from build123d import *

# Parameters (mm, degrees)
F0_W      = 9
F0_H      = 10
F0_W_2    = 44
F0_H_2    = 16
F0_W_3    = 7
F0_R      = 1
F1_DEPTH  = 0.5
F3_R      = 0.5
F3_W      = 0.3535533906
F3_H      = 10
F4_DEPTH  = 0.5
F6_R      = 0.5
F6_W      = 0.3535533906
F6_H      = 10
F7_DEPTH  = 0.5
F8_R      = 1.25
F9_DEPTH  = 0.5
F10_R     = 1.25
F11_DEPTH = 0.5
F12_DEPTH = 0.5
F14_DEPTH = 15
F13_W     = 2
F13_H     = 14.5
F15_DEPTH = 1
F16_W     = 2
F16_H     = 1
F17_DEPTH = 1
F18_W     = 1
F18_H     = 29.75
F19_DEPTH = 6.5
F21_D     = 2.5
F21_DEPTH = 8
F21_TIP   = 0.7510757738
F23_DEPTH = 1
F25_DEPTH = 1
F26_R     = 1.25
F27_DEPTH = 1
F28_W     = 5
F28_H     = 1
F29_DEPTH = 5
F30_DEPTH = 14.25
F31_W     = 5
F31_H     = 4
F31_H_2   = 1
F32_DEPTH = 1
F34_DEPTH = 0.5
F35_W     = 1
F35_H     = 42
F36_DEPTH = 0.5
F38_DEPTH = 0.5
F39_W     = 0.5
F39_H     = 42
F39_W_2   = 1
F40_DEPTH = 0.5


# Not quite as in the source:
# - a feature of the source that left no trace in its solid (it failed there, or was rolled back) is left out
# - a feature names something its author has since deleted; it is built from what else it names


with BuildPart() as f1:
    # F0 (on Front) → F1 (new body)
    with BuildSketch(Plane.XZ):
        with Locations((-25.5, 0)):
            Rectangle(F0_W, F0_H)
        with Locations((1, 13)):
            Rectangle(F0_W_2, F0_H_2)
        with Locations((1, 0)):
            Rectangle(F0_W_2, F0_H)
        with Locations((26.5, 0)):
            Rectangle(F0_W_3, F0_H)
        with Locations((1, -13)):
            Rectangle(F0_W_2, F0_H_2)
        with Locations((1, -13)):
            Circle(F0_R, mode=Mode.SUBTRACT)
    extrude(amount=F1_DEPTH)

    # F3 (on face) → F4 (join)
    with BuildSketch(Plane(origin=(15, 15, 0), x_dir=(0.7071067812, -0.7071067812, 0), z_dir=(-0.7071067812, -0.7071067812, 0))):
        with BuildLine():
            Line((21.5667568262, 5), (21.5667568262, -5))
            Line((21.5667568262, -5), (32.2132034356, -5))
            ThreePointArc((32.2132034356, -5), (32.9203102168, -4.7071067812), (33.2132034356, -4))
            Line((33.2132034356, -4), (33.2132034356, 4))
            ThreePointArc((33.2132034356, 4), (32.9203102168, 4.7071067812), (32.2132034356, 5))
            Line((32.2132034356, 5), (21.5667568262, 5))
        make_face()
        with Locations((23.2132034356, -2)):
            Circle(F3_R, mode=Mode.SUBTRACT)
        with Locations((23.2132034356, 0)):
            Circle(F3_R, mode=Mode.SUBTRACT)
        with Locations((23.2132034356, 2)):
            Circle(F3_R, mode=Mode.SUBTRACT)
        with Locations((21.3899801309, 0)):
            Rectangle(F3_W, F3_H)
    extrude(amount=F4_DEPTH)

    # F6 (on face) → F7 (join)
    with BuildSketch(Plane(origin=(-15, 15, 0), x_dir=(0.7071067812, 0.7071067812, 0), z_dir=(0.7071067812, -0.7071067812, 0))):
        with BuildLine():
            Line((-21.5667568262, -5), (-21.5667568262, 5))
            Line((-21.5667568262, 5), (-32.2132034356, 5))
            ThreePointArc((-32.2132034356, 5), (-32.9203102168, 4.7071067812), (-33.2132034356, 4))
            Line((-33.2132034356, 4), (-33.2132034356, -4))
            ThreePointArc((-33.2132034356, -4), (-32.9203102168, -4.7071067812), (-32.2132034356, -5))
            Line((-32.2132034356, -5), (-21.5667568262, -5))
        make_face()
        with Locations((-22.2132034356, -2)):
            Circle(F6_R, mode=Mode.SUBTRACT)
        with Locations((-22.2132034356, 0)):
            Circle(F6_R, mode=Mode.SUBTRACT)
        with Locations((-22.2132034356, 2)):
            Circle(F6_R, mode=Mode.SUBTRACT)
        with Locations((-21.3899801309, 0)):
            Rectangle(F6_W, F6_H)
    extrude(amount=F7_DEPTH)

    # F8 (on face) → F9 (join)
    with BuildSketch(Plane(origin=(15, 15, 0), x_dir=(-0.7071067812, 0.7071067812, 0), z_dir=(0.7071067812, 0.7071067812, 0))):
        with Locations((-30.7632034356, 0)):
            Circle(F8_R)
    extrude(amount=F9_DEPTH)

    # F10 (on face) → F11 (join)
    with BuildSketch(Plane(origin=(-15, 15, 0), x_dir=(-0.7071067812, -0.7071067812, 0), z_dir=(-0.7071067812, 0.7071067812, 0))):
        with Locations((30.7632034356, 0)):
            Circle(F10_R)
    extrude(amount=F11_DEPTH)

    # F0 (on Front) → F12 (join)
    with BuildSketch(Plane.XZ):
        with Locations((1, 13)):
            Rectangle(F0_W_2, F0_H_2)
        with Locations((1, -13)):
            Rectangle(F0_W_2, F0_H_2)
        with Locations((1, -13)):
            Circle(F0_R, mode=Mode.SUBTRACT)
    extrude(amount=F12_DEPTH)

    # F0 (on Front) → F14 (join)
    with BuildSketch(Plane.XZ):
        with Locations((1, -13)):
            Circle(F0_R)
    extrude(amount=F14_DEPTH)

    # F13 (on face) → F15 (join)
    with BuildSketch(Plane(origin=(0, 0, -21), x_dir=(1, 0, 0), z_dir=(0, 0, -1))):
        with Locations((-20, 7.75)):
            Rectangle(F13_W, F13_H)
        with Locations((22, 7.75)):
            Rectangle(F13_W, F13_H)
    extrude(amount=-F15_DEPTH)

    # F16 (on face) → F17 (join)
    with BuildSketch(Plane.XZ.offset(15)):
        with BuildLine():
            Line((-19, -21), (-21, -21))
            Line((-21, -21), (-21, -42.75))
            Line((-21, -42.75), (23, -42.75))
            Line((23, -42.75), (23, -21))
            Line((23, -21), (21, -21))
            Line((21, -21), (21, -20))
            Line((21, -20), (23, -20))
            Line((23, -20), (23, -13))
            Line((23, -13), (2, -13))
            ThreePointArc((2, -13), (1, -14), (0, -13))
            Line((0, -13), (-21, -13))
            Line((-21, -13), (-21, -20))
            Line((-21, -20), (-19, -20))
            Line((-19, -20), (-19, -21))
        make_face()
        with Locations((-20, -20.5)):
            Rectangle(F16_W, F16_H)
        with BuildLine():
            ThreePointArc((2, -13), (1, -12), (0, -13))
            Line((0, -13), (2, -13))
        make_face()
        with BuildLine():
            Line((2, -13), (0, -13))
            ThreePointArc((0, -13), (1, -14), (2, -13))
        make_face()
        with Locations((22, -20.5)):
            Rectangle(F16_W, F16_H)
    extrude(amount=F17_DEPTH)

    # F18 (on face) → F19 (join)
    with BuildSketch(Plane.XZ.offset(16)):
        with Locations((1, -27.875)):
            Rectangle(F18_W, F18_H)
    extrude(amount=F19_DEPTH)

    # F21
    with Locations(Plane.YZ.offset(1.5)):
        with Locations((-19.25, -39)):
            Hole(F21_D / 2, depth=F21_DEPTH)
            with Locations((0, 0, -(F21_DEPTH + F21_TIP / 2))):  # 118° drill point
                Cone(0, F21_D / 2, F21_TIP, mode=Mode.SUBTRACT)

    # F22 (on face) → F23 (join)
    with BuildSketch(Plane(origin=(0, 0, -42.75), x_dir=(1, 0, 0), z_dir=(0, 0, -1))):
        Polygon((-21, 15), (23, 15), (23, 16), (1.5, 16), (1.5, 22.5), (0.5, 22.5), (0.5, 16), (-21, 16), align=None)
    extrude(amount=F23_DEPTH)

    # F22 (on face) → F25 (join)
    with BuildSketch(Plane(origin=(0, 0, -42.75), x_dir=(1, 0, 0), z_dir=(0, 0, -1))):
        Polygon((1.5, 16), (23, 16), (23, 51.5), (18, 51.5), (18, 52.5), (23, 52.5), (23, 53), (23, 90), (-21, 90), (-21, 52.5), (-16, 52.5), (-16, 51.5), (-21, 51.5), (-21, 16), (0.5, 16), (0.5, 22.5), (1.5, 22.5), align=None)
        Polygon((-21, 15), (23, 15), (23, 16), (1.5, 16), (1.5, 22.5), (0.5, 22.5), (0.5, 16), (-21, 16), align=None)
    extrude(amount=F25_DEPTH)

    # F26 (on face) → F27 (join)
    with BuildSketch(Plane.XZ.offset(90)):
        Polygon((-16, -43.75), (-21, -43.75), (-21, -58), (-21, -70.1), (-16, -70.1), align=None)
        with Locations((-18.5, -67.075)):
            Circle(F26_R, mode=Mode.SUBTRACT)
        Polygon((23, -43.75), (18, -43.75), (18, -70.1), (23, -70.1), (23, -58), align=None)
        with Locations((20.5, -67.075)):
            Circle(F26_R, mode=Mode.SUBTRACT)
    extrude(amount=-F27_DEPTH)

    # F28 (on face) → F29 (join)
    with BuildSketch(Plane(origin=(0, -89, 0), x_dir=(-1, 0, 0), z_dir=(0, 1, 0))):
        with Locations((18.5, -57.5)):
            Rectangle(F28_W, F28_H)
        with Locations((-20.5, -57.5)):
            Rectangle(F28_W, F28_H)
    extrude(amount=F29_DEPTH)

    # F22 (on face) → F30 (join)
    with BuildSketch(Plane(origin=(0, 0, -42.75), x_dir=(1, 0, 0), z_dir=(0, 0, -1))):
        Polygon((-21, 52), (-21, 51.5), (-16, 51.5), (-16, 52.5), (-21, 52.5), align=None)
        Polygon((18, 51.5), (23, 51.5), (23, 52), (23, 52.5), (18, 52.5), align=None)
    extrude(amount=F30_DEPTH)

    # F31 (on face) → F32 (join)
    with BuildSketch(Plane(origin=(0, 0, -57), x_dir=(1, 0, 0), z_dir=(0, 0, -1))):
        with Locations((20.5, 49.5)):
            Rectangle(F31_W, F31_H)
        with Locations((20.5, 52)):
            Rectangle(F31_W, F31_H_2)
        with Locations((-18.5, 49.5)):
            Rectangle(F31_W, F31_H)
        with Locations((-18.5, 52)):
            Rectangle(F31_W, F31_H_2)
    extrude(amount=F32_DEPTH)

    # F33 (on face) → F34 (join)
    with BuildSketch(Plane.YZ.offset(23)):
        Polygon((0, 21), (0, 5), (0, -5), (0, -21), (1.5, -21), (1.5, 21), align=None)
    extrude(amount=-F34_DEPTH)

    # F35 (on face) → F36 (join)
    with BuildSketch(Plane(origin=(0, 1.5, 0), x_dir=(-1, 0, 0), z_dir=(0, 1, 0))):
        with Locations((-22, 0)):
            Rectangle(F35_W, F35_H)
    extrude(amount=-F36_DEPTH)

    # F37 (on face) → F38 (join)
    with BuildSketch(Plane(origin=(-21, 0, 0), x_dir=(0, -1, 0), z_dir=(-1, 0, 0))):
        Polygon((-1.5, -21), (0, -21), (0, -5), (0, 21), (-1.5, 21), align=None)
    extrude(amount=-F38_DEPTH)

    # F39 (on face) → F40 (join)
    with BuildSketch(Plane(origin=(0, 1.5, 0), x_dir=(-1, 0, 0), z_dir=(0, 1, 0))):
        with Locations((20.75, 0)):
            Rectangle(F39_W, F39_H)
        with Locations((20, 0)):
            Rectangle(F39_W_2, F39_H)
    extrude(amount=F40_DEPTH)


solid = f1.part
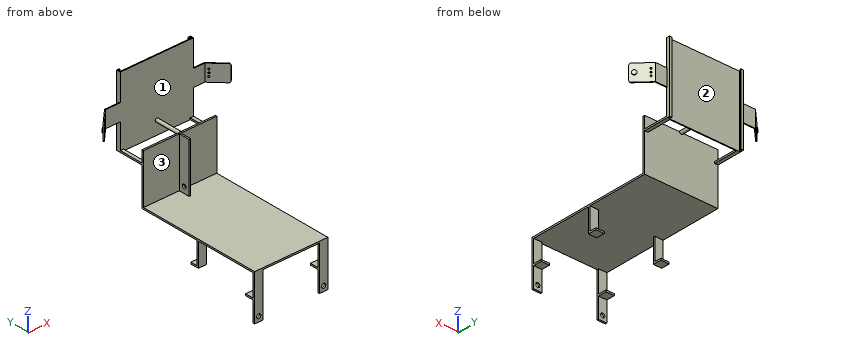
The listing builds one solid part. Answer for the finished solid, in the listing's coordinates (mm). Face numbers are marked on the shaded views. Coordinates: 2 decimals unless noted, no trailing zeros. Order: outer loops, then holes, each group sorted by start corner. A loop starts at its lowest first (then second) coordinate and runs counter-clockwise, first axis right, second up. Notation, with made-up numbers: (15, 72) -> (55, 72) arc R31 ccw to (55, 103) -> close; hole circle Ø7 at (85, 68). An arc over 180 degrees is marked (long way). Answer in a Markdown table with one row per item. Add a question column.
Item 1: Find the intervals of material crossed by L1, parallel to Z at x = 20.5, y = -89.2 (3 decimals); L2, parallel to Y at x = -14.5, z = -13.5; L3, parallel to Z at x = 0.8, y = -19.25, in increasing order. Write a range as from..to.
Item 2: Find section D-D (z = 12.5). Write down the section's boundary in (x, y), then the cut area to 4 significant figures.
Item 3: Find section C-C (x = 8). Write down the section's boundary in (y, z).
Item 4: Each of these flat-tipped pins is pushed along its axis until it touches: P1, Ø12, axis at x = 22.5, y = -61.5, coming from the -Z side; P2, Ø12.5, axis at x = 10.5, z = -1.5, coming from the -Y side; P3, Ø2.5, axis at x = 20.5, y = -85.5, coming from the +Z side. Where does it stop, or does it pass through?
Item 5: Find section B-B (y = -19.25). Write down the section's boundary in (x, z), then the cut area to 4 significant figures.
Item 6: Determine the mould class of the marked faces 1, 2 and 3 for opening direction X: +X half, -X half, draft (parallel to the pull), parting line (faces both ways), or undercut.
Item 7: Find section A-A (z = -39). Write down the section's boundary in (x, y), then the cut area to 3 significant figures.
Result set:
| question | item | result |
|---|---|---|
| 1 | L1 | z = -70.1..-68.325, -65.825..-42.75 |
| 1 | L2 | y = -16..-15, -0.5..0 |
| 1 | L3 | z = -43.75..-40.25, -37.75..-13 |
| 2 | outline | (-21, -0.5) -> (23, -0.5) -> (23, 1.5) -> (21.5, 1.5) -> (21.5, 1) -> (22.5, 1) -> (22.5, 0) -> (-20.5, 0) -> (-20.5, 1.5) -> (-19.5, 1.5) -> (-19.5, 2) -> (-21, 2) -> close |
| 2 | area | 24.75 mm² |
| 3 | outline | (-90, -43.75) -> (-15, -43.75) -> (-15, -13) -> (-16, -13) -> (-16, -42.75) -> (-90, -42.75) -> close; (-0.5, -21) -> (0, -21) -> (0, 21) -> (-0.5, 21) -> close |
| 4 | P1 | stops at z = -43.75 |
| 4 | P2 | stops at y = -0.5 |
| 4 | P3 | stops at z = -42.75 |
| 5 | outline | (-21, -43.75) -> (23, -43.75) -> (23, -42.75) -> (1.5, -42.75) -> (1.5, -40.25) -> (0.5, -40.25) -> (0.5, -42.75) -> (-21, -42.75) -> close; (0.5, -37.75) -> (1.5, -37.75) -> (1.5, -13) -> (0.5, -13) -> close |
| 5 | area | 71.25 mm² |
| 6 | face 1 | undercut |
| 6 | face 2 | undercut |
| 6 | face 3 | draft |
| 7 | outline | (-21, -16) -> (0.5, -16) -> (0.5, -18) -> (1.5, -18) -> (1.5, -16) -> (23, -16) -> (23, -15) -> (-21, -15) -> close; (0.5, -22.5) -> (1.5, -22.5) -> (1.5, -20.5) -> (0.5, -20.5) -> close |
| 7 | area | 48.0 mm² |
